For this review, take the finished solid that the model builds, in its own axes (mm). A direction names the side the tool comes from. Round coordinates to 2 decimals unless told otherwise and drop trailing zeros. Order: outer loops, then holes, each group sorted by start corner. A loop starts at its lowest first (then second) coordinate and runs counter-clockwise, first axis right, second up. Notation, with made-up numbers: M 72.5,-5.5 L 119.5,-5.5 A29 ccw 119.5,18.5 Z; hole C 65,62.25 d10. An arc over 180 degrees is marked long. Write item = value, one per line. Start each with the question number.
from build123d import *

# Parameters (mm, degrees)
HOLE_WIZARD_M101_D           = 8.5
HOLE_WIZARD_M101_DEPTH       = 24.946342369
HOLE_WIZARD_M101_CSINK_D     = 10.05
HOLE_WIZARD_M101_CSINK_ANGLE = 90
HOLE_WIZARD_M101_TIP         = 2.553657631
CUT_EXTRUDE_1_DEPTH          = 15


with BuildPart() as part:
    # Эскиз1 → Повернуть1 (revolve)
    with BuildSketch(Plane.XY):
        Polygon((0, 0), (0, 15), (1, 16), (15, 16), (15, 24), (16, 25), (19, 25), (20, 24), (20, 10), (170, 10), (171, 9), (171, 7.5), (173, 7.5), (173, 8), (174, 9), (183, 9), (184, 8), (184, 7.5), (203, 7.5), (204, 6.5), (204, 5), (216, 5), (216, 4), (216, 0), align=None)
    revolve(axis=Axis((0, 0, 0), (1, 0, 0)))

    # Отверстие обработанное метчиком M101
    with Locations(Plane.ZY):
        with Locations((0, 0)):
            CounterSinkHole(HOLE_WIZARD_M101_D / 2, HOLE_WIZARD_M101_CSINK_D / 2, depth=HOLE_WIZARD_M101_DEPTH, counter_sink_angle=HOLE_WIZARD_M101_CSINK_ANGLE)
            with Locations((0, 0, -(HOLE_WIZARD_M101_DEPTH + HOLE_WIZARD_M101_TIP / 2))):  # 118° drill point
                Cone(0, HOLE_WIZARD_M101_D / 2, HOLE_WIZARD_M101_TIP, mode=Mode.SUBTRACT)

    # Эскиз5 → Вырез-Вытянуть1 (cut)
    with BuildSketch(Plane(origin=(216, 0, 0), x_dir=(0, 0, -1), z_dir=(1, 0, 0))):
        Polygon((3.464101615, 0), (1.732050808, 3), (-1.732050808, 3), (-3.464101615, 0), (-1.732050808, -3), (1.732050808, -3), align=None)
    extrude(amount=-CUT_EXTRUDE_1_DEPTH, mode=Mode.SUBTRACT)


solid = part.part
(1) We need section B-B, the plane x = 66. Write out the cut boundary in (y, z), then the cut area to 3 significant figures.
(2) We need section A-A, the plane x = 177. Write out the cut boundary in (y, z).
(3) For faces 4 (the flat face through (20, 10.3, 0.3)), 5 (the flat face through (171, -2, 7.4)), 6 (the flat face through (216, -3.3, 0.1)), 7 (the cylindrical face through (8.1, -3.47, -15.62)), list the 3-axis set-ups (+Z, -Z, +X, -X, +Y, -Y) from which the entire face can be reached by the end or side of a thin tool; tool diameter is ignored.
(4) Insertion check: pin 1 (4 mm diameter, centred on x = 65.5, z = 2.5, fed in from -Y); pin 2 (10 mm diameter, centred on x = 149, y = 5, fed in from -Z); pin 3 (3 mm diameter, centred on x = 142, z = 9, fed in from -Y). Each pin has a flat end and moves straight along its axis. Give the tip position at first contact, or say it passes through.
(5) Draft analysis for pull direction Y (two halves, no side actions). For faces 1 (the cylindrical face through (13.03, 3.584, -2.285)), 2 (the cylindrical face through (178.563, -1.172, 8.923)), 3 (the flat face through (173, -5, -6)), state which applies: released by +Y, released by -Y, zero draft, split by the parting line, or undercut.
(6) For line 1 along Z through (x, y) = (9.25, 0); line 2 along Z through (x, y) = (17, 0); line 3 along X through (y, z) = (-7.5, -10), list the stretches that pass through material, from the lowest coordinate up.
Values:
q1.outline = C 0,0 d20
q1.area = 314 mm²
q2.outline = C 0,0 d18
q3.face_4 = +X
q3.face_5 = none
q3.face_6 = +Z, -Z, +X, +Y, -Y
q3.face_7 = -X
q4.pin_1 = -9.99
q4.pin_2 = -10
q4.pin_3 = -6.61
q5.face_1 = undercut
q5.face_2 = split by the parting line
q5.face_3 = zero draft
q6.line_1 = -16 to -4.25, 4.25 to 16
q6.line_2 = -25 to -4.25, 4.25 to 25
q6.line_3 = 0 to 20
